Can you work these out from the drawing? Everything is in mm from the part's minimum corner. A direction names the side the tool comes from. Give positions to 0.01 mm unless a question says otherwise; leave off trailing zeros. Loops run counter-clockwise (first coordinate to the right, second up) from the corner with the lowest first, then second, coordinate; pieces in that order, holes last. Notation, with made-up numbers: (11, -35) - (24, -35) arc R25 cw to (24, -16) - close; hole circle Ø7 at (-22, 68.25). An arc over 180 degrees is marked (long way). Write each question's results on one line, items separated by ' | '. Start each with the question number.
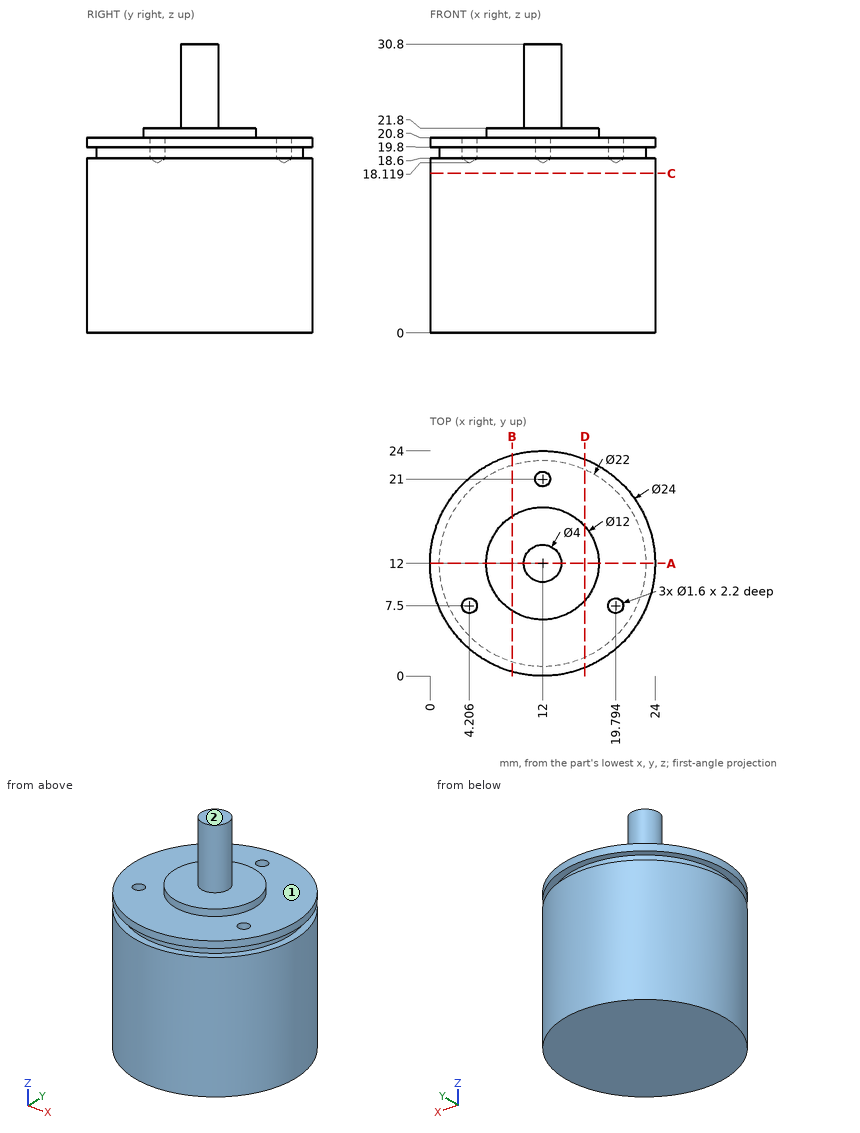
Q1. Which directions (+Z, -Z, +X, -X, +Y, -Y) give clear straight access to the entire face, cutting with the end or side of a thin tool? Please do the marked faces 1 and 2.
Q2. I want a section at B-B, the plane x = 8.75. List the corners of the cut face in (y, z) for me.
Q3. I want a section at D-D, the plane x = 16.5. List the corners of the cut face in (y, z) for me, then the cut area to 3 significant figures.
Q4. I'm going to push flat-ended pins straight in: pin 1 Ø1.4 at (x, y) = (19.79, 7.5) entering from +Z; pin 2 Ø1.5 at (y, z) = (17, 14.5) entering from -X; pin 3 Ø3 at (x, z) = (6, 4.5) entering from -Y (1 decimal). Where does each tip first touch, or does it pass through?
Q5. I need wall thicknesses on L1, parallel to Y at x = 12, z = 19.9; L2, parallel to X at y = 7.5, z = 19.95 (1 decimal); L3, parallel to X at y = 7.5, z = 19.1 (1 decimal). Which ranges of each line are inside material? Lowest first, please. Write a range as from..to.
Q6. I want a section at C-C, the plane z = 17. List the corners of the cut face in (x, y) for me.
Q7. I want a section at A-A, the plane y = 12. List the corners of the cut face in (x, z) for me.
Conclusion:
1) face 1: +Z | face 2: +Z, +X, -X, +Y, -Y
2) outline: (0.45, 0) - (23.55, 0) - (23.55, 18.6) - (22.51, 18.6) - (22.51, 19.8) - (23.55, 19.8) - (23.55, 20.8) - (17.04, 20.8) - (17.04, 21.8) - (6.96, 21.8) - (6.96, 20.8) - (0.45, 20.8) - (0.45, 19.8) - (1.49, 19.8) - (1.49, 18.6) - (0.45, 18.6) - close
3) outline: (0.88, 0) - (23.12, 0) - (23.12, 18.6) - (22.04, 18.6) - (22.04, 19.8) - (23.12, 19.8) - (23.12, 20.8) - (15.97, 20.8) - (15.97, 21.8) - (8.03, 21.8) - (8.03, 20.8) - (0.88, 20.8) - (0.88, 19.8) - (1.96, 19.8) - (1.96, 18.6) - (0.88, 18.6) - close | area: 468 mm^2
4) pin 1: z = 18.54 | pin 2: x = 0.78 | pin 3: y = 0.9
5) L1: 0..20.2, 21.8..24 | L2: 0.9..3.4, 5..19, 20.6..23.1 | L3: 2..3.4, 5..19, 20.6..22
6) outline: circle Ø24 at (12, 12)
7) outline: (0, 0) - (24, 0) - (24, 18.6) - (23, 18.6) - (23, 19.8) - (24, 19.8) - (24, 20.8) - (18, 20.8) - (18, 21.8) - (14, 21.8) - (14, 30.8) - (10, 30.8) - (10, 21.8) - (6, 21.8) - (6, 20.8) - (0, 20.8) - (0, 19.8) - (1, 19.8) - (1, 18.6) - (0, 18.6) - close
